Here's the drawing with two shaded views (mm, measured from the low corner). I have some questions. Round coordinates to 2 decimals unless told otherwise and drop trailing zeros. Loops run counter-clockwise (first coordinate to the right, second up) from the corner with the lowest first, then second, coordinate; pieces in that order, holes last. Notation, with made-up numbers: M 36,71.5 L 92,71.5 A21 cw 92,104.5 Z; hole C -7.5,74.5 d11. An arc over 180 degrees is marked long. Answer as a JSON object with one key per item and string values.
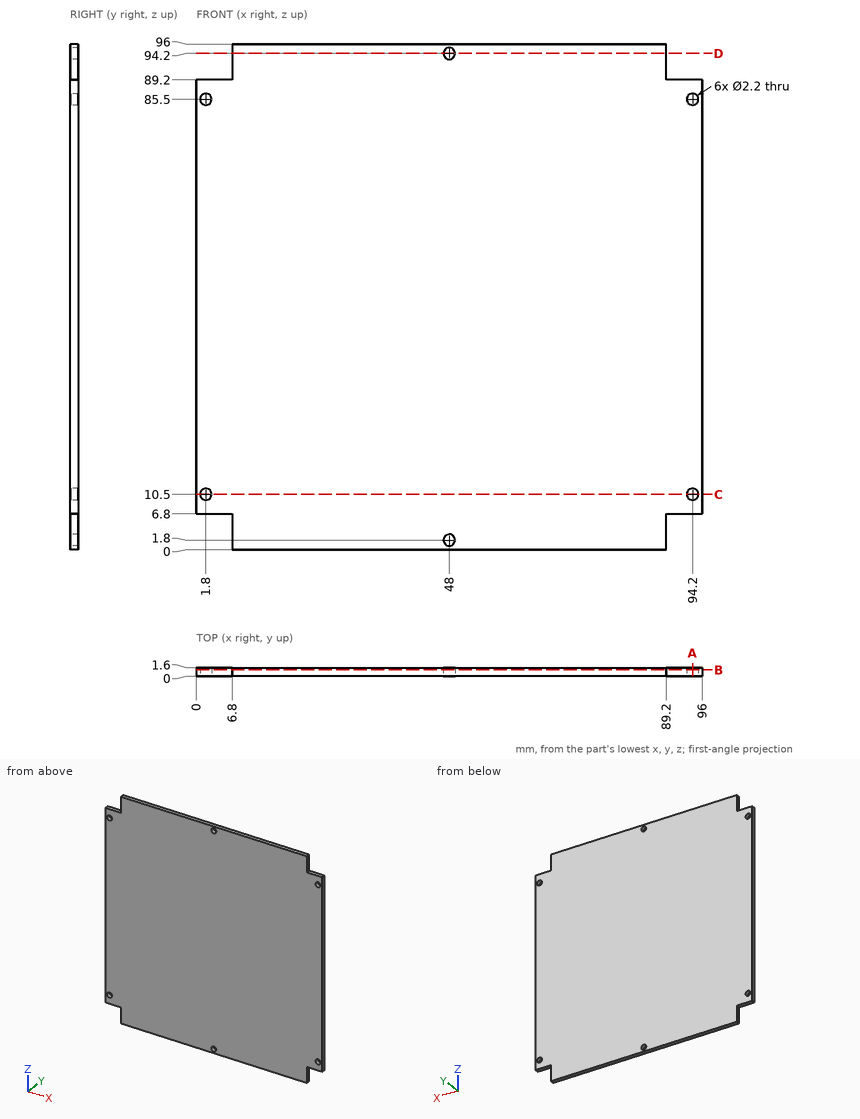
Item 1: I want a section at B-B on y = 1.15. List the corners of the cut face in (x, z) for me, plus the area to 3 significant figures.
Solution:
{"outline": "M 0,6.8 L 6.8,6.8 L 6.8,0 L 89.2,0 L 89.2,6.8 L 96,6.8 L 96,89.2 L 89.2,89.2 L 89.2,96 L 6.8,96 L 6.8,89.2 L 0,89.2 Z; hole C 1.8,10.5 d2.2; hole C 1.8,85.5 d2.2; hole C 48,1.8 d2.2; hole C 48,94.2 d2.2; hole C 94.2,10.5 d2.2; hole C 94.2,85.5 d2.2", "area": "9,010 mm2"}
Item 2: I want a section at A-A on x = 94.2. List the corners of the cut face in (y, z) for me, plus the area to 3 significant figures.
Solution:
{"outline": "M 0,6.8 L 1.6,6.8 L 1.6,9.4 L 0,9.4 Z; M 0,11.6 L 1.6,11.6 L 1.6,84.4 L 0,84.4 Z; M 0,86.6 L 1.6,86.6 L 1.6,89.2 L 0,89.2 Z", "area": "125 mm2"}
Item 3: I want a section at D-D on z = 94.2. List the corners of the cut face in (x, y) for me, plus the area to 3 significant figures.
Solution:
{"outline": "M 6.8,0 L 46.9,0 L 46.9,1.6 L 6.8,1.6 Z; M 49.1,0 L 89.2,0 L 89.2,1.6 L 49.1,1.6 Z", "area": "128 mm2"}
Item 4: I want a section at C-C on z = 10.5. List the corners of the cut face in (x, y) for me.
Solution:
{"outline": "M 0,0 L 0.7,0 L 0.7,1.6 L 0,1.6 Z; M 2.9,0 L 93.1,0 L 93.1,1.6 L 2.9,1.6 Z; M 95.3,0 L 96,0 L 96,1.6 L 95.3,1.6 Z"}
Item 5: If I drill on L1, parallel to X at y = 0.5, z = 85.5; L2, parallel to Z at x = 94.2, y = 1.15, over which ranges is the centre line in solid material (lowest first)? Write a range as from..to.
Solution:
{"L1": "x = 0..0.7, 2.9..93.1, 95.3..96", "L2": "z = 6.8..9.4, 11.6..84.4, 86.6..89.2"}
Item 6: For P1, Ø0.5, axis at y = 0.5, z = 3, coming from the +X side; P2, Ø0.8, axis at y = 1, z = 93.5, coming from the -X side; P3, Ø0.5, axis at x = 92.5, y = 1, coming from the +Z side, each with a flat end and sliding along its axis, tell me the tip position at first contact or that it passes through.
Solution:
{"P1": "stops at x = 89.2", "P2": "stops at x = 6.8", "P3": "stops at z = 89.2"}
